Geometry check sheet. Reference: the model listing, model coordinates, mm. Face numbers are marked on the shaded views. A direction names the side the tool comes from. Round coordinates to 2 decimals unless told otherwise and drop trailing zeros. Order: outer loops, then holes, each group sorted by start corner. A loop starts at its lowest first (then second) coordinate and runs counter-clockwise, first axis right, second up.
(1) Sectioned sample at B-B (z = -146.5). Record the boundary of the cut face in (x, y), plus the area to 3 significant figures.
(2) Set-up check for the marked faces 1, 2, 3 and 4: record each of +Z, -Z, +X, -X, +Y, -Y from which the full face is reachable in a straight line by a thin tool's end or side.
(3) Release check for a two-part mould opening along X. For the marked faces 5, 6 and 7 record: +X half, -X half, draft (parallel to the pull), parting line (faces both ways), or undercut.
(4) Material ranges on line 1 along Y through (x, z) = (-383, -110); line 2 along X through (y, z) = (888, -17); line 3 along Y through (x, z) = (-425.5, -98), recorded low to high.
(5) Go/stop test with flat-tipped pins: pin 1 (2 mm diameter, centred on y = 875, z = -45.5, fed in from +X); pin 2 (12 mm diameter, centred on y = 425, z = -177, fed in from -X); pin 3 (1 mm diameter, centred on y = 747, z = -37, fed in from +X). Record where each tip stops, or that it passes through.
(6) Sectioned sample at D-D (x = -464.5). Record the boundary of the cut face in (y, z).
(7) Sectioned sample at C-C (y = 885). Record the boundary of the cut face in (x, z), plus the area to 3 significant figures.
(8) Sectioned sample at A-A (x = -250). Record the boundary of the cut face in (y, z), plus the area to 3 significant figures.
from build123d import *

# Parameters (mm, degrees)
F1_DEPTH = 10
F2_DEPTH = 800
F4_DEPTH = 10
F5_W     = 345.459491
F5_H     = 265.73801
F6_DEPTH = 300


with BuildPart() as f1:
    # F0 (on Front) → F1 (new body)
    with BuildSketch(Plane.XZ):
        with BuildLine():
            ThreePointArc((-500, 0), (-250, -250), (0, 0))
            Line((0, 0), (-10, 0))
            ThreePointArc((-10, 0), (-250, -239.685813), (-490, 0))
            Line((-490, 0), (-500, 0))
        make_face()
        with BuildLine():
            ThreePointArc((-490, 0), (-250, -239.685813), (-10, 0))
            Line((-10, 0), (-490, 0))
        make_face()
    extrude(amount=F1_DEPTH)

    # F0 (on Front) → F2 (join)
    with BuildSketch(Plane.XZ):
        with BuildLine():
            ThreePointArc((-500, 0), (-250, -250), (0, 0))
            Line((0, 0), (-10, 0))
            ThreePointArc((-10, 0), (-250, -239.685813), (-490, 0))
            Line((-490, 0), (-500, 0))
        make_face()
    extrude(amount=-F2_DEPTH)

    # F3 (on face) → F4 (join)
    with BuildSketch(Plane(origin=(0, 800, 0), x_dir=(-1, 0, 0), z_dir=(0, 1, 0))):
        with BuildLine():
            Line((490, 0), (10, 0))
            ThreePointArc((10, 0), (250, -239.685813), (490, 0))
        make_face()
    extrude(amount=-F4_DEPTH)

    # F5 (on face) → F6 (join)
    with BuildSketch(Plane(origin=(0, 800, 0), x_dir=(-1, 0, 0), z_dir=(0, 1, 0))):
        with Locations((242.526159, -99.256635)):
            Rectangle(F5_W, F5_H)
    extrude(amount=F6_DEPTH)


solid = f1.part
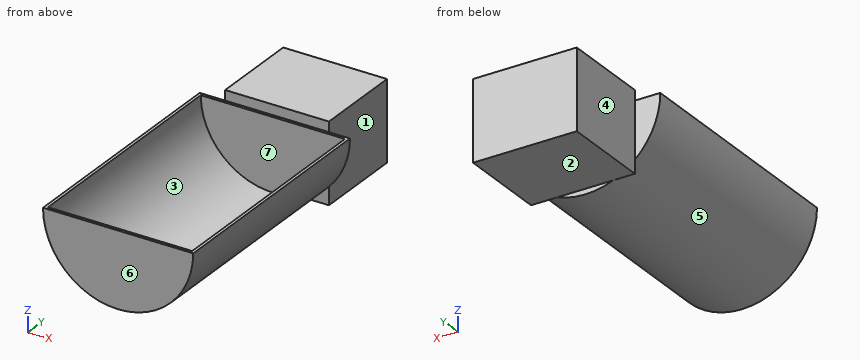
Answer below:
1. outline: (-452.58, -10) - (-47.42, -10) - (-47.42, 800) - (-69.8, 800) - (-69.8, 1100) - (-415.26, 1100) - (-415.26, 800) - (-452.58, 800) - close; hole (-439.86, 0) - (-60.14, 0) - (-60.14, 790) - (-439.86, 790) - close
1. area: 132,000 mm2
2. face 1: +Z, -Z, +X, +Y
2. face 2: -Z, +X, -X, +Y
2. face 3: +Z
2. face 4: +Z, -Z, -X, +Y
3. face 5: parting line
3. face 6: draft
3. face 7: undercut
4. line 1: y = -10 to 0, 790 to 1100
4. line 2: x = -415.26 to -69.8
4. line 3: y = -10 to 0, 790 to 800
5. pin 1: stops at x = -69.8
5. pin 2: stops at x = -432.37
5. pin 3: stops at x = -2.68
6. outline: (-10, -128.41) - (800, -128.41) - (800, 0) - (790, 0) - (790, -107.34) - (0, -107.34) - (0, 0) - (-10, 0) - close
7. outline: (-415.26, -232.13) - (-69.8, -232.13) - (-69.8, 33.61) - (-415.26, 33.61) - close
7. area: 91,800 mm2
8. outline: (-10, -250) - (800, -250) - (800, -232.13) - (1100, -232.13) - (1100, 33.61) - (800, 33.61) - (800, 0) - (790, 0) - (790, -239.69) - (0, -239.69) - (0, 0) - (-10, 0) - close
8. area: 92,900 mm2
